from build123d import *

# Parameters (mm, degrees)
SKETCH1_W           = 70
SKETCH1_H           = 35
BOSS_EXTRUDE1_DEPTH = 50
SHELL1_T            = -3
SKETCH2_W           = 50
SKETCH2_H           = 70
BOSS_EXTRUDE2_DEPTH = 3
SKETCH4_R           = 6.5
BOSS_EXTRUDE3_DEPTH = 6
CUT_EXTRUDE1_REACH  = 46
SKETCH5_R           = 4.5
SKETCH6_W           = 50
SKETCH6_H           = 3
BOSS_EXTRUDE4_DEPTH = 10
SKETCH8_R           = 3.2
CUT_EXTRUDE3_DEPTH  = 4
SKETCH9_R           = 3.2
CUT_EXTRUDE4_DEPTH  = 4
FILLET1_R           = 10
FILLET2_R           = 10


with BuildPart() as part:
    # Sketch1 → Boss-Extrude1 (new body)
    with BuildSketch(Plane(origin=(0, 0, 0), x_dir=(0, 0, -1), z_dir=(1, 0, 0))):
        Rectangle(SKETCH1_W, SKETCH1_H)
    extrude(amount=BOSS_EXTRUDE1_DEPTH)

    # Shell1
    shell1_openings = [part.faces().sort_by_distance(p)[0] for p in [
        (25, 17.5, 0),
    ]]
    offset(amount=SHELL1_T, openings=shell1_openings, kind=Kind.INTERSECTION)

    # Sketch2 → Boss-Extrude2 (add)
    with BuildSketch(Plane(origin=(0, 17.5, 0), x_dir=(1, 0, 0), z_dir=(0, 1, 0))):
        with Locations((25, 0)):
            Rectangle(SKETCH2_W, SKETCH2_H)
    extrude(amount=BOSS_EXTRUDE2_DEPTH)

    # Sketch4 → Boss-Extrude3 (add)
    with BuildSketch(Plane.XZ.offset(17.5)):
        with Locations((25, 0)):
            Circle(SKETCH4_R)
    extrude(amount=BOSS_EXTRUDE3_DEPTH)

    # Sketch5 → Cut-Extrude1 (cut, up to next)
    with BuildSketch(Plane.XZ.offset(23.5), mode=Mode.PRIVATE) as cut_extrude1_sk1:
        with Locations((25, 0)):
            Circle(SKETCH5_R)
    cut_extrude1_tool1 = extrude(cut_extrude1_sk1.sketch, amount=-CUT_EXTRUDE1_REACH, mode=Mode.PRIVATE) & part.part
    add(cut_extrude1_tool1.solids().sort_by_distance((25, -23.5, 0))[0], mode=Mode.SUBTRACT)

    # Sketch6 → Boss-Extrude4 (add)
    with BuildSketch(Plane.XY.offset(35)):
        with Locations((25, 19)):
            Rectangle(SKETCH6_W, SKETCH6_H)
    extrude(amount=BOSS_EXTRUDE4_DEPTH)

    # Sketch8 → Cut-Extrude3 (cut, through all)
    with BuildSketch(Plane.XZ.offset(-17.5)):
        with Locations((12.3, 40)):
            Circle(SKETCH8_R)
    extrude(amount=-CUT_EXTRUDE3_DEPTH, mode=Mode.SUBTRACT)

    # Sketch9 → Cut-Extrude4 (cut, through all)
    with BuildSketch(Plane.XZ.offset(-17.5)):
        with Locations((37.7, 40)):
            Circle(SKETCH9_R)
    extrude(amount=-CUT_EXTRUDE4_DEPTH, mode=Mode.SUBTRACT)

    # Fillet1
    fillet1_edges = [part.edges().sort_by_distance(p)[0] for p in [
        (50, -17.5, 0),
        (50, 1.5, -35),
        (0, -17.5, 0),
        (0, 0, 35),
        (50, 0, 35),
        (0, 1.5, -35),
        (25, -17.5, -35),
        (25, -17.5, 35),
    ]]
    fillet(fillet1_edges, radius=FILLET1_R)

    # Fillet2
    fillet2_edges = [part.edges().sort_by_distance(p)[0] for p in [
        (3, 1.5, -32),
        (25, -14.5, -32),
        (3, 1.5, 32),
        (3, -14.5, 0),
        (25, -14.5, 32),
        (47, 1.5, -32),
        (47, 1.5, 32),
        (47, -14.5, 0),
    ]]
    fillet(fillet2_edges, radius=FILLET2_R)


solid = part.part
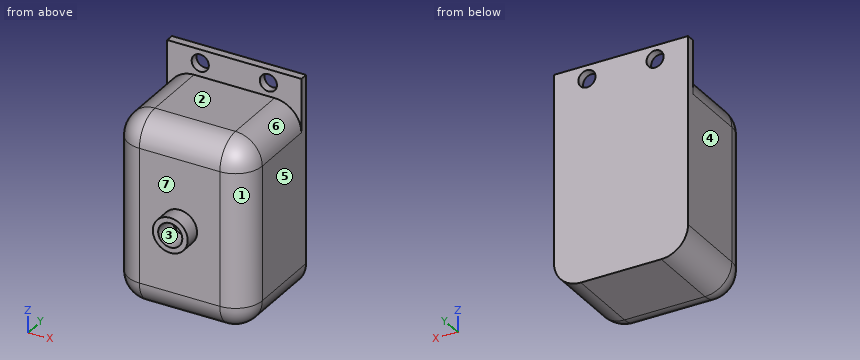
Source: CAD feature listing. Evaluate the final solid. Frame: model axes, mm. Face numbers are marked on the shaded views. A direction names the side the tool comes from. Give positions to 0.01 mm unless a question says otherwise; leave off trailing zeros. Order: outer loops, then holes, each group sorted by start corner. A loop starts at its lowest first (then second) coordinate and runs counter-clockwise, first axis right, second up. Notation, with made-up numbers: (62, -5) -> (82, -5) arc R22 cw to (82, 22) -> close; hole circle Ø9 at (51, -26.5). An arc over 180 degrees is marked (long way). Use a Markdown table: item, result.
1) Section query D-D, the plane x = 25. Return the cut outline in (y, z).
Answer list:
| item | result |
|---|---|
| outline | (-23.5, -6.5) -> (-17.5, -6.5) -> (-17.5, -25) arc R10 ccw to (-7.5, -35) -> (20.5, -35) -> (20.5, 45) -> (17.5, 45) -> (17.5, 35) -> (-7.5, 35) arc R10 ccw to (-17.5, 25) -> (-17.5, 6.5) -> (-23.5, 6.5) -> (-23.5, 4.5) -> (-14.5, 4.5) -> (-14.5, 22) arc R10 cw to (-4.5, 32) -> (17.5, 32) -> (17.5, -32) -> (-4.5, -32) arc R10 cw to (-14.5, -22) -> (-14.5, -4.5) -> (-23.5, -4.5) -> close |
2) Ray query, line 1 along Z through (x, y) = (25, -19); line 2 along Z through (x, y) = (35.5, 0); line 3 along Y through (x, z) = (35, 0). Return the intervals inside material, ascending. Write a range as [from, to].
Answer list:
| item | result |
|---|---|
| line 1 | [-6.5, -4.5], [4.5, 6.5] |
| line 2 | [-35, -32], [32, 35] |
| line 3 | [-17.5, -14.5], [17.5, 20.5] |
3) Contact query for flat-ended pins moving along their axis: P1, Ø2, axis at y = -15.5, z = -13.5, coming from the -X side; P2, Ø20, axis at x = 29.5, y = 5.5, coming from the +Z side; P3, Ø8, axis at y = -18, z = -8, coming from the -X side. Output: stop coordinate, or through.
Answer list:
| item | result |
|---|---|
| P1 | x = 2.86 |
| P2 | z = 35 |
| P3 | x = 2.4 |
4) Reachability of the marked faces 5, 6 and 7 from +Z, -Z, +X, -X, +Y, -Y: full face, straight path, thin tool, end or side. Return the list, or none.
Answer list:
| item | result |
|---|---|
| face 5 | +Z, -Z, +X, +Y, -Y |
| face 6 | +Z, +X, -Y |
| face 7 | -Y |
5) Section query B-B, the plane y = -2.5. Return the cut outline in (x, z), then the cut area to 3 significant figures.
Answer list:
| item | result |
|---|---|
| outline | (0, -25) arc R10 ccw to (10, -35) -> (40, -35) arc R10 ccw to (50, -25) -> (50, 25) arc R10 ccw to (40, 35) -> (10, 35) arc R10 ccw to (0, 25) -> close; hole (3, -22) arc R10 ccw to (13, -32) -> (37, -32) arc R10 ccw to (47, -22) -> (47, 22) arc R10 ccw to (37, 32) -> (13, 32) arc R10 ccw to (3, 22) -> close |
| area | 684 mm² |
6) Section query C-C, the plane z = 8.5. Return the cut outline in (x, y).
Answer list:
| item | result |
|---|---|
| outline | (0, -7.5) arc R10 ccw to (10, -17.5) -> (40, -17.5) arc R10 ccw to (50, -7.5) -> (50, 20.5) -> (0, 20.5) -> close; hole (3, -4.5) arc R10 ccw to (13, -14.5) -> (37, -14.5) arc R10 ccw to (47, -4.5) -> (47, 17.5) -> (3, 17.5) -> close |
7) Section query A-A, the plane z = 40. Return the cut outline in (x, y).
Answer list:
| item | result |
|---|---|
| outline | (0, 17.5) -> (9.1, 17.5) -> (9.1, 20.5) -> (0, 20.5) -> close; (15.5, 17.5) -> (34.5, 17.5) -> (34.5, 20.5) -> (15.5, 20.5) -> close; (40.9, 17.5) -> (50, 17.5) -> (50, 20.5) -> (40.9, 20.5) -> close |
8) Mould query, pull axis X, two halves, no side actions, for the marked faces 1, 2, 3 and 4. Classes: +X half, -X half, draft (parallel to the pull), parting line (faces both ways), or undercut.
Answer list:
| item | result |
|---|---|
| face 1 | +X half |
| face 2 | draft |
| face 3 | undercut |
| face 4 | -X half |
